Source: CAD feature listing. Evaluate the final solid. Frame: model axes, mm. Face numbers are marked on the shaded views. A direction names the side the tool comes from. Coordinates: 2 decimals unless noted, no trailing zeros. Write each loop counter-clockwise with the first axis right and the second up, starting at its lowest first coordinate (ties: lowest second). Pieces come first, ordered by that corner, then holes. Notation, with made-up numbers: M -2,-38.75 L 12,-38.75 A28 ccw 12,-16.75 Z; hole C 35,70 d3. An arc over 180 degrees is marked long. Write item = value, one per line. Start each with the question number.
1. Line query: line 1 along Y through (x, z) = (13.98, -0.4); line 2 along X through (y, z) = (11, -0.5); line 3 along Y through (x, z) = (13.98, -0.95). Output: solid intervals per line, ascending.
2. Pin query (flat end, axial travel): pin 1 Ø0.8 at (y, z) = (20.5, 9) entering from +X; pin 2 Ø0.8 at (x, y) = (2, 21) entering from +Z; pin 3 Ø2.5 at (x, y) = (13.98, 9.65) entering from -Z; pin 4 Ø3 at (x, y) = (13.5, 4) entering from +Z. Return the tip coordinate at first contact, or that it passes through.
3. Section query B-B (y = 3.65). Output: boundary loops of the cut face in (x, z), then the cut area to 3 significant figures.
4. Access query for the marked faces 1 and 2. Directions: +Z, -Z, +X, -X, +Y, -Y. A direction counts if a zero-diameter tool reaches every point of the face in a straight line with its end or side. Return the directions, or none.
5. Section query C-C (x = 16.5). Output: boundary loops of the cut face in (y, z), then the cut area to 3 significant figures.
6. Section query D-D (z = -0.5). Output: boundary loops of the cut face in (x, y).
7. Section query A-A (z = 7.78). Output: boundary loops of the cut face in (x, y), then the cut area to 3 significant figures.
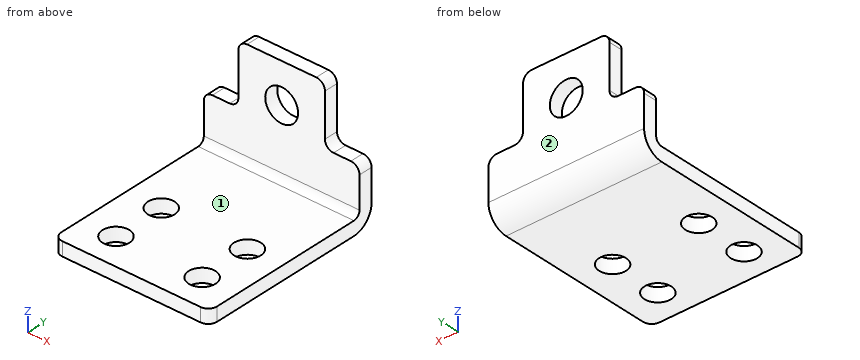
```python
from build123d import *

# Parameters (mm, degrees)
SKETCH2_W                    = 18
SKETCH2_H                    = 21.5
BASE_FLANGE1_DEPTH           = 1.6
EDGE_FLANGE1_STRIP_W         = 7.8732
EDGE_FLANGE1_STRIP_H         = 1.6
EDGE_FLANGE1_STRIP_CUT_DEPTH = 18
EDGE_FLANGE1_DEPTH           = 18
SKETCH10_R                   = 1.9
SKETCH10_W                   = 4
SKETCH10_H                   = 7
CUT_EXTRUDE1_DEPTH           = 10
FILLET1_R                    = 1
SKETCH11_R                   = 1.5494
CUT_EXTRUDE2_DEPTH           = 10


# Sheet-metal steps are written as plain solids
with BuildPart() as part:
    # Sketch2 → Base-Flange1 (new body)
    with BuildSketch(Plane.XY):
        with Locations((9, 10.75)):
            Rectangle(SKETCH2_W, SKETCH2_H)
    extrude(amount=-BASE_FLANGE1_DEPTH)

    # Edge-Flange1 strip (across the edge) → Edge-Flange1 strip cut (cut)
    with BuildSketch(Plane(origin=(18, 21.5, 0), x_dir=(0, -1, 0), z_dir=(-1, 0, 0))):
        with Locations((-1.6, -0.8)):
            Rectangle(EDGE_FLANGE1_STRIP_W, EDGE_FLANGE1_STRIP_H)
    extrude(amount=EDGE_FLANGE1_STRIP_CUT_DEPTH, mode=Mode.SUBTRACT)

    # Edge-Flange1 section (across the edge) → Edge-Flange1 (add)
    with BuildSketch(Plane(origin=(18, 21.5, 0), x_dir=(0, -1, 0), z_dir=(-1, 0, 0))):
        with BuildLine():
            Line((0, 0.7366), (0, 12.4))
            Line((0, 12.4), (1.6, 12.4))
            Line((1.6, 12.4), (1.6, 0.7366))
            ThreePointArc((1.6, 0.7366), (1.815745145, 0.215745145), (2.3366, 0))
            Line((2.3366, 0), (2.3366, -1.6))
            ThreePointArc((2.3366, -1.6), (0.684374295, -0.915625705), (0, 0.7366))
        make_face()
    extrude(amount=EDGE_FLANGE1_DEPTH)

    # Sketch10 → Cut-Extrude1 (cut)
    with BuildSketch(Plane(origin=(0, 21.5, 0), x_dir=(1, 0, 0), z_dir=(0, 1, 0))):
        with Locations(Location((9, -7.78, 0), (0, 0, 270))):
            Circle(SKETCH10_R)
        with Locations((2, -8.9)):
            Rectangle(SKETCH10_W, SKETCH10_H)
        with Locations((16, -8.9)):
            Rectangle(SKETCH10_W, SKETCH10_H)
    extrude(amount=-CUT_EXTRUDE1_DEPTH, mode=Mode.SUBTRACT)

    # Fillet1
    fillet1_edges = [part.edges().sort_by_distance(p)[0] for p in [
        (0, 0, -0.8),
        (18, 0, -0.8),
        (0, 20.7, 5.4),
        (18, 20.7, 5.4),
        (4, 20.7, 5.4),
        (14, 20.7, 5.4),
        (14, 20.7, 12.4),
        (4, 20.7, 12.4),
    ]]
    fillet(fillet1_edges, radius=FILLET1_R)

    # Sketch11 → Cut-Extrude2 (cut)
    with BuildSketch(Plane.XY):
        with Locations((4.02, 9.65)):
            Circle(SKETCH11_R)
        with Locations((13.98, 9.65)):
            Circle(SKETCH11_R)
        with Locations((4.02, 3.65)):
            Circle(SKETCH11_R)
        with Locations((13.98, 3.65)):
            Circle(SKETCH11_R)
    extrude(amount=-CUT_EXTRUDE2_DEPTH, mode=Mode.SUBTRACT)


solid = part.part
```
Results are:
q1.line_1 = 0 to 2.1, 5.2 to 8.1, 11.2 to 21.2
q1.line_2 = 0 to 3.26, 4.78 to 13.22, 14.74 to 18
q1.line_3 = 0 to 2.1, 5.2 to 8.1, 11.2 to 20.78
q2.pin_1 = 14
q2.pin_2 = 5.4
q2.pin_3 = through
q2.pin_4 = 0
q3.outline = M 0,-1.6 L 2.47,-1.6 L 2.47,0 L 0,0 Z; M 5.57,-1.6 L 12.43,-1.6 L 12.43,0 L 5.57,0 Z; M 15.53,-1.6 L 18,-1.6 L 18,0 L 15.53,0 Z
q3.area = 18.9 mm^2
q4.face_1 = +Z, +X, -X, -Y
q4.face_2 = +Z, -Z, +X, -X, +Y
q5.outline = M 0,-1.6 L 19.16,-1.6 A2.34 ccw 21.5,0.74 L 21.5,5.4 L 19.9,5.4 L 19.9,0.74 A0.74 cw 19.16,0 L 0,0 Z
q5.area = 42.0 mm^2
q6.outline = M 0,1 A1 ccw 1,0 L 17,0 A1 ccw 18,1 L 18,21.15 L 0,21.15 Z; hole C 4.02,3.65 d3.1; hole C 4.02,9.65 d3.1; hole C 13.98,3.65 d3.1; hole C 13.98,9.65 d3.1
q7.outline = M 4,19.9 L 7.1,19.9 L 7.1,21.5 L 4,21.5 Z; M 10.9,19.9 L 14,19.9 L 14,21.5 L 10.9,21.5 Z
q7.area = 9.92 mm^2
